Check sheet for the modelled part. Datum: model origin and axes. Units: mm. Face numbers are marked on the shaded views. Give positions to 0.01 mm unless a question says otherwise; leave off trailing zeros. Write each loop counter-clockwise with the first axis right and the second up, starting at its lowest first coordinate (ties: lowest second). Pieces come first, ordered by that corner, then holes. Notation, with made-up numbers: (82.25, 31.25) -> (117.25, 31.25) arc R13 ccw to (117.25, 38.25) -> close; hole circle Ø10 at (72.5, 74.25). An arc over 180 degrees is marked (long way). Answer as a JSON object with one key per item and string values.
from build123d import *

# Parameters (mm, degrees)
SKETCH1_W           = 21
SKETCH1_H           = 15
BOSS_EXTRUDE1_DEPTH = 2
SKETCH2_R           = 2.25
CUT_EXTRUDE1_DEPTH  = 14.057564857
FILLET1_R           = 2


with BuildPart() as part:
    # Sketch1 → Boss-Extrude1 (new body)
    with BuildSketch(Plane.XY):
        Rectangle(SKETCH1_W, SKETCH1_H)
    extrude(amount=-BOSS_EXTRUDE1_DEPTH)

    # Sketch2 → Cut-Extrude1 (cut, through all)
    with BuildSketch(Plane.XY):
        Circle(SKETCH2_R)
    extrude(amount=-CUT_EXTRUDE1_DEPTH, mode=Mode.SUBTRACT)

    # Fillet1
    fillet1_edges = [part.edges().sort_by_distance(p)[0] for p in [
        (10.5, -7.5, -1),
        (-10.5, -7.5, -1),
        (-10.5, 7.5, -1),
        (10.5, 7.5, -1),
    ]]
    fillet(fillet1_edges, radius=FILLET1_R)


solid = part.part
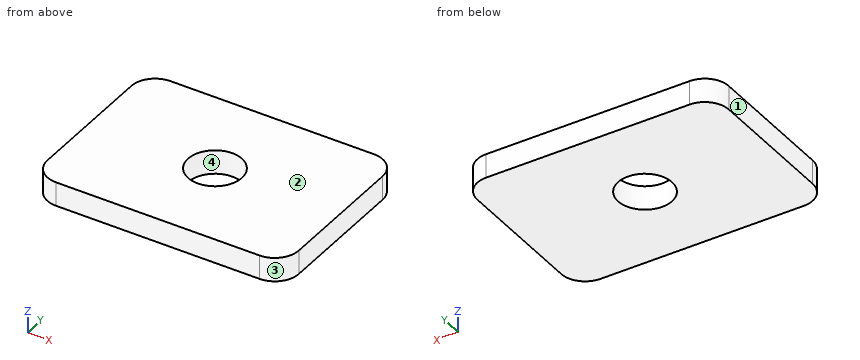
1. Sectioned sample at A-A, the plane y = 0. Enter the section's corners in (x, z).
Determined:
{"outline": "(-10.5, -2) -> (-2.25, -2) -> (-2.25, 0) -> (-10.5, 0) -> close; (2.25, -2) -> (10.5, -2) -> (10.5, 0) -> (2.25, 0) -> close"}
2. Scan lines: L1, parallel to Y at x = 0, z = -1.35; L2, parallel to X at y = -1, z = -0.05; L3, parallel to Y at x = -0.75, z = -1.55. Record each from-to range of solid material in increasing order. Write a range as [from, to].
Determined:
{"L1": "[-7.5, -2.25], [2.25, 7.5]", "L2": "[-10.5, -2.02], [2.02, 10.5]", "L3": "[-7.5, -2.12], [2.12, 7.5]"}
3. Sectioned sample at C-C, the plane x = 0. Enter the section's corners in (y, z), plus the area to 3 significant figures.
Determined:
{"outline": "(-7.5, -2) -> (-2.25, -2) -> (-2.25, 0) -> (-7.5, 0) -> close; (2.25, -2) -> (7.5, -2) -> (7.5, 0) -> (2.25, 0) -> close", "area": "21.0 mm^2"}
4. Sectioned sample at B-B, the plane z = -1. Enter the section's corners in (x, y), plus the area to 3 significant figures.
Determined:
{"outline": "(-10.5, -5.5) arc R2 ccw to (-8.5, -7.5) -> (8.5, -7.5) arc R2 ccw to (10.5, -5.5) -> (10.5, 5.5) arc R2 ccw to (8.5, 7.5) -> (-8.5, 7.5) arc R2 ccw to (-10.5, 5.5) -> close; hole circle Ø4.5 at (0, 0)", "area": "296 mm^2"}
5. Mould release check, pull along X, two halves, no side actions. Record for the marked faces 1, 2, 3 and 4: released by +X, released by -X, zero draft, split by the parting line, or undercut.
Determined:
{"face 1": "released by -X", "face 2": "zero draft", "face 3": "released by +X", "face 4": "undercut"}
